CAD build for the part. Positions are in the model's coordinates, mm. A direction names the side the tool comes from. Coordinates: 2 decimals unless noted, no trailing zeros. Order: outer loops, then holes, each group sorted by start corner. A loop starts at its lowest first (then second) coordinate and runs counter-clockwise, first axis right, second up.
from build123d import *

# Parameters (mm, degrees)
F0_W     = 105.362009
F0_H     = 60.93785
F1_DEPTH = 88.9
F2_W     = 35.585844
F2_H     = 31.86445
F3_DEPTH = 25.4


with BuildPart() as f1:
    # F0 (on Front) → F1 (new body)
    with BuildSketch(Plane.XZ):
        with Locations((4.070277, 0.697763)):
            Rectangle(F0_W, F0_H)
    extrude(amount=F1_DEPTH)

    # F2 (on face) → F3 (join)
    with BuildSketch(Plane.XZ.offset(88.9)):
        Rectangle(F2_W, F2_H)
    extrude(amount=F3_DEPTH)


solid = f1.part
1) Drill centre lines: probe 1 along Y at (x, z) = (22, -23); probe 2 along X at (y, z) = (-93.5, 13.5). Where is each one in solid material? Low to high.
2) Which spindle directions (+Z, -Z, +X, -X, +Y, -Y) get a long thin tool onto all of the face, cutting with end or side? Do faces 1 (the flat face through (-17.793, -101, 0)), 2 (the flat face through (17.793, -101, 0)), 3 (the flat face through (0, -101, -15.932)), 4 (the flat face through (0, -101, 15.932)). Say none if no direction does.
3) Pin check, flat tips, straight feed: P1, Ø12.5, axis at y = -98.5, z = -5, coming from the -X side; P2, Ø7.5, axis at y = -101.5, z = 2.5, coming from the +X side; P3, Ø1.5, axis at x = -15, y = -96.5, coming from the -Z side. Stop position of each tip, or through.
4) Slice it at B-B (z = 12). List the corners of the cut face in (x, y), plus the area to 3 significant figures.
5) Slice it at C-C (x = 30.5). List the corners of the cut face in (y, z).
6) Slice it at D-D (z = -26). List the corners of the cut face in (x, y).
7) Slice it at A-A (x = 1.5). List the corners of the cut face in (y, z), plus the area to 3 significant figures.
Worked out:
1. probe 1: y = -88.9 to 0
1. probe 2: x = -17.79 to 17.79
2. face 1: +Z, -Z, -X, -Y
2. face 2: +Z, -Z, +X, -Y
2. face 3: -Z, +X, -X, -Y
2. face 4: +Z, +X, -X, -Y
3. P1: stops at x = -17.79
3. P2: stops at x = 17.79
3. P3: stops at z = -15.93
4. outline: (-48.61, -88.9) - (-17.79, -88.9) - (-17.79, -114.3) - (17.79, -114.3) - (17.79, -88.9) - (56.75, -88.9) - (56.75, 0) - (-48.61, 0) - close
4. area: 10,300 mm2
5. outline: (-88.9, -29.77) - (0, -29.77) - (0, 31.17) - (-88.9, 31.17) - close
6. outline: (-48.61, -88.9) - (56.75, -88.9) - (56.75, 0) - (-48.61, 0) - close
7. outline: (-114.3, -15.93) - (-88.9, -15.93) - (-88.9, -29.77) - (0, -29.77) - (0, 31.17) - (-88.9, 31.17) - (-88.9, 15.93) - (-114.3, 15.93) - close
7. area: 6,230 mm2
